Autodesk Inventor part; units mm, degrees
ref_plane "YZ Plane" through (0, 0, 0) normal (1, 0, 0) x (0, 1, 0)
ref_plane "XZ Plane" through (0, 0, 0) normal (0, 1, 0) x (-1, 0, 0)
ref_plane "XY Plane" through (0, 0, 0) normal (0, 0, 1) x (1, 0, 0)
sketch "Sketch1" plane through (0, 0, 0) normal (0, 0, 1) x (1, 0, 0)
  line L0 (2.8868, 0) -> (1.4434, -2.5)
  line L1 (1.4434, -2.5) -> (-1.4434, -2.5)
  line L2 (-1.4434, -2.5) -> (-2.8868, 0)
  line L3 (-2.8868, 0) -> (-1.4434, 2.5)
  line L4 (-1.4434, 2.5) -> (1.4434, 2.5)
  line L5 (1.4434, 2.5) -> (2.8868, 0)
  point P0 (0, 0)
  point P1 (0, 0)
  dimension "d0" = 5
extrude "Extrusion1" add sketch "Sketch1" along normal blind 5
sketch "Sketch3" plane through (0, 0, 0) normal (0, 0, -1) x (-1, 0, 0)
  circle A0 centre (0, 0) radius 1.25
  dimension "d6" = 2.5
extrude "Extrusion3" cut sketch "Sketch3" against normal through all
sketch "Sketch4" plane through (0, 0, 5) normal (0, 0, 1) x (1, 0, 0)
  circle A0 centre (0, 0) radius 1.25
  dimension "d9" = 2.5
extrude "Extrusion4" add sketch "Sketch4" along normal blind 6
sketch "Sketch5" plane through (0, 0, 5) normal (0, 0, -1) x (-1, 0, 0)
  circle A0 centre (0, 0) radius 1.25
extrude "Extrusion5" add sketch "Sketch5" along normal blind 3
properties part number "M2.5x6mm_Standoff_ 971050154"
Can you work these out from the model? Positions are in its coordinate system, mm. A direction names the side the tool comes from. Coordinates: 2 decimals unless noted, no trailing zeros. Write each loop counter-clockwise with the first axis right and the second up, starting at its lowest first coordinate (ties: lowest second). Pieces come first, ordered by that corner, then holes. Notation, with made-up numbers: (71.5, -27.75) - (130.5, -27.75) arc R19 ccw to (130.5, 3.25) - close; hole circle Ø1 at (82, 1). An arc over 180 degrees is marked (long way). Return JSON: item names as keys, results as strings.
Q1. If we section it at B-B (x = 0): Please give me the cut outline in (y, z), then the cut area to 3 significant figures.
Computed values:
{"outline": "(-2.5, 0) - (-1.25, 0) - (-1.25, 2) - (1.25, 2) - (1.25, 0) - (2.5, 0) - (2.5, 5) - (1.25, 5) - (1.25, 11) - (-1.25, 11) - (-1.25, 5) - (-2.5, 5) - close", "area": "35.0 mm2"}
Q2. If we section it at D-D (z = 4): Please give me the cut outline in (x, y).
Computed values:
{"outline": "(-2.89, 0) - (-1.44, -2.5) - (1.44, -2.5) - (2.89, 0) - (1.44, 2.5) - (-1.44, 2.5) - close"}
Q3. I'm going to push flat-ended pins straight in: pin 1 Ø1 at (x, y) = (0.5, 0) entering from -Z; pin 2 Ø3 at (y, z) = (1, 7.5) entering from +X. Where does each tip first touch, or does it pass through?
Computed values:
{"pin 1": "stops at z = 2", "pin 2": "stops at x = 1.25"}
Q4. Thinking about a two-plate mould opening in X: for faces 4 (the flat face through (2.175, -1.233, 2.465)), 5 (the flat face through (0, 0, 11)), 6 (the cylindrical face through (0.27, -1.22, 0.99)), which applies, +X half, -X half, draft (parallel to the pull), parting line (faces both ways), or undercut?
Computed values:
{"face 4": "+X half", "face 5": "draft", "face 6": "undercut"}
Q5. If we section it at A-A (z = 1): Please give me the cut outline in (x, y), then the cut area to 3 significant figures.
Computed values:
{"outline": "(-2.89, 0) - (-1.44, -2.5) - (1.44, -2.5) - (2.89, 0) - (1.44, 2.5) - (-1.44, 2.5) - close; hole circle Ø2.5 at (0, 0)", "area": "16.7 mm2"}
Q6. If we section it at C-C (y = -0.75): Please give me the cut outline in (x, z).
Computed values:
{"outline": "(-2.45, 0) - (-1, 0) - (-1, 2) - (1, 2) - (1, 0) - (2.45, 0) - (2.45, 5) - (1, 5) - (1, 11) - (-1, 11) - (-1, 5) - (-2.45, 5) - close"}
Q7. On a 3-axis mill with a long thin cutter (end or side, diameter ignored), from which of +Z, -Z, +X, -X, +Y, -Y can I reach the whole of each face in a straight line? I mean faces 1 (the flat face through (0, 0, 2)), 2 (the flat face through (-2.155, -1.267, 2.465)), 3 (the cylindrical face through (-0.27, 1.22, 7.96)). Say none if no direction works.
Computed values:
{"face 1": "-Z", "face 2": "+Z, -Z, -X, -Y", "face 3": "+Z"}
Q8. Please list where these lines run through material, in increasing order: L1, parallel to Y at x = 0, z = 1.55; L2, parallel to Z at x = 0.65, y = -1.35; L3, parallel to Z at x = -0.5, y = 0.35. Write a range as from..to.
Computed values:
{"L1": "y = -2.5..-1.25, 1.25..2.5", "L2": "z = 0..5", "L3": "z = 2..11"}
